Geometry: final body of the model. Coordinates: model frame, mm. Give positions to 0.01 mm unless a question says otherwise; leave off trailing zeros. Order: outer loops, then holes, each group sorted by start corner. A loop starts at its lowest first (then second) coordinate and runs counter-clockwise, first axis right, second up. Notation, with made-up numbers: (-15, 9) -> (20, 9) arc R22 ccw to (20, 46) -> close; hole circle Ø6 at (-35, 40). An arc over 180 degrees is marked (long way). Answer in a Markdown table with one row per item. Add a question column.
Q1. Contact query for flat-ended pins moving along their axis: P1, Ø6, axis at x = 14, z = 14.5, coming from the +Y side; P2, Ø4, axis at x = 56, z = 12.5, coming from the +Y side. Output: stop coordinate, or through.
Q2. Line query: line 1 along X through (y, z) = (597, 1.5); line 2 along X through (y, z) = (457.5, 7.5); line 3 along Y through (x, z) = (69.5, 15). Output: solid intervals per line, ascending. Write a range as from..to.
Q3. Cut plane C-C on x = 105.5. Return the cut outline in (y, z) (3 decimals).
Q4. Cut plane B-B on y = 529.5. Return the cut outline in (x, z), and give its area (3 significant figures).
Q5. Cut plane A-A on z = 3. Return the cut outline in (x, y), and give its area (3 significant figures).
from build123d import *

# Parameters (mm, degrees)
F1_DEPTH = 19.05
F2_R     = 254
F3_R     = 25.4
F5_DEPTH = 139.701


with BuildPart() as f1:
    # F0 (on Top) → F1 (new body)
    with BuildSketch(Plane.XY):
        Polygon((0, 666.75), (0, 0), (139.7, 0), (139.7, 381), (88.9, 666.75), align=None)
    extrude(amount=F1_DEPTH)

    # F2
    f2_edges = [f1.edges().sort_by_distance(p)[0] for p in [
        (139.7, 381, 9.525),
    ]]
    fillet(f2_edges, radius=F2_R)

    # F3
    f3_edges = [f1.edges().sort_by_distance(p)[0] for p in [
        (139.7, 0, 9.525),
    ]]
    fillet(f3_edges, radius=F3_R)

    # F4 (on face) → F5 (cut, through all)
    with BuildSketch(Plane(origin=(0, 0, 0), x_dir=(0, -1, 0), z_dir=(-1, 0, 0))):
        Polygon((-663.390971, 0), (-666.75, 19.05), (-666.75, 0), align=None)
    extrude(amount=-F5_DEPTH, mode=Mode.SUBTRACT)


solid = f1.part
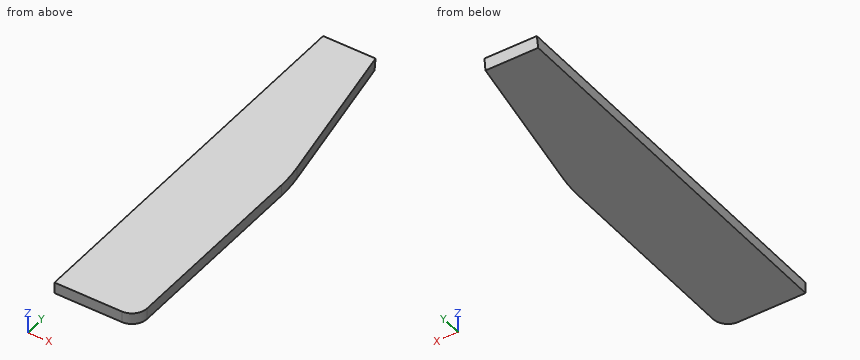
Completed:
| question | item | result |
|---|---|---|
| 1 | P1 | stops at y = 666.48 |
| 1 | P2 | stops at y = 665.95 |
| 2 | line 1 | x = 0..101.3 |
| 2 | line 2 | x = 0..126.1 |
| 2 | line 3 | y = 0..666.04 |
| 3 | outline | (0, 0) -> (573.375, 0) -> (573.375, 19.05) -> (0, 19.05) -> close |
| 4 | outline | (0, 0) -> (113.3, 0) -> (113.3, 19.05) -> (0, 19.05) -> close |
| 4 | area | 2,160 mm² |
| 5 | outline | (0, 0) -> (114.3, 0) arc R25.4 ccw to (139.7, 25.4) -> (139.7, 358.6) arc R254 ccw to (135.78, 403.06) -> (89.4, 663.92) -> (0, 663.92) -> close |
| 5 | area | 85,500 mm² |
